Work out the finished part from the listing and answer in its coordinate system (mm). Round coordinates to 2 decimals unless told otherwise and drop trailing zeros. Order: outer loops, then holes, each group sorted by start corner. A loop starts at its lowest first (then second) coordinate and runs counter-clockwise, first axis right, second up. Notation, with made-up numbers: (5, 74.5) - (41, 74.5) arc R14 ccw to (41, 92.5) - close; hole circle Ø9 at (64, -29.5). An arc over 180 degrees is marked (long way). Answer in a Markdown table with one row per item.
Autodesk Inventor part; units mm, degrees
ref_plane "Start Plane" through (0, 0, 19.7356) normal (0, 0, 1) x (1, 0, 0)
ref_plane "End Plane" through (0, 0, 1295.0132) normal (0, 0, 1) x (1, 0, 0)
ref_plane "Work Plane4" through (-472.3083, -9, 221.6126) normal (-0.3985724, 0, -0.9171369) x (-0.9171369, 0, 0.3985724)
ref_plane "Start Plane" through (0, 0, 19.7356) normal (0, 0, 1) x (1, 0, 0)
ref_plane "End Plane" through (0, 0, 1295.0132) normal (0, 0, 1) x (1, 0, 0)
sketch "Sketch" plane through (0, 0, 0) normal (0, 0, 1) x (1, 0, 0)
  line L0 (-15, -9) -> (-15, 9)
  line L1 (-9, 15) -> (9, 15)
  line L2 (15, 9) -> (15, -9)
  line L3 (9, -15) -> (-9, -15)
  arc A0 (-15, -9) -> (-9, -15) centre (-9, -9) ccw
  arc A1 (-9, 15) -> (-15, 9) centre (-9, 9) ccw
  arc A2 (15, 9) -> (9, 15) centre (9, 9) ccw
  arc A3 (9, -15) -> (15, -9) centre (9, -9) ccw
  arc A4 (-9, 12) -> (-12, 9) centre (-9, 9) ccw
  line L4 (-9, 12) -> (9, 12)
  arc A5 (12, 9) -> (9, 12) centre (9, 9) ccw
  line L5 (12, 9) -> (12, -9)
  arc A6 (9, -12) -> (12, -9) centre (9, -9) ccw
  line L6 (9, -12) -> (-9, -12)
  arc A7 (-12, -9) -> (-9, -12) centre (-9, -9) ccw
  line L7 (-12, -9) -> (-12, 9)
  line L8 (0, 22.7397) -> (0, -22.7397) construction
  line L9 (-22.7397, 0) -> (22.7397, 0) construction
  dimension "d7" = 6
  dimension "d10" = 30
  dimension "d11" = 30
  dimension "d12" = 3
  dimension "d15" = 15
  dimension "d16" = 15
extrude "Body" add sketch "Sketch" along normal up to surface (1275.2776 mm away) from surface at 19.7356
sketch "Sketch3" plane through (0, 0, 0) normal (0, 0, 1) x (1, 0, 0)
  line L0 (0, 0) -> (10, 0)
ref_plane "Work Plane3" through (0, 0, 0) normal (0, -1, 0) x (1, 0, 0)
ref_plane "Work Plane4" through (-472.3083, -9, 221.6126) normal (-0.3985724, 0, -0.9171369) x (-0.9171369, 0, 0.3985724)
split "Split1" plane through (-472.3083, -9, 221.6126) removes the side toward (-0.3985724, 0, -0.9171369)
ref_plane "Work Plane5" through (-464.5298, 9, 201.8769) normal (-0.9171369, 0, 0.3985724) x (0.3985724, 0, 0.9171369)
split "Split2" plane through (-464.5298, 9, 201.8769) removes the side toward (-0.9171369, 0, 0.3985724)
ref_plane "Work Plane6" through (1.6776, 9, 1293.5139) normal (-0.1118382, 0, 0.9937264) x (0.9937264, 0, 0.1118382)
split "Split3" plane through (1.6776, 9, 1293.5139) removes the side toward (-0.1118382, 0, 0.9937264)
ref_plane "Work Plane7" through (584.1015, 9, 1381.6839) normal (0.9171369, 0, -0.3985724) x (-0.3985724, 0, -0.9171369)
split "Split4" plane through (584.1015, 9, 1381.6839) removes the side toward (0.9171369, 0, -0.3985724)
sketch "Sketch4" plane through (0, 0, 0) normal (0, -1, 0) x (1, 0, 0)
  line L0 (-2, 19.7356) -> (12, 19.7356)
  line L1 (-2, 1295.0132) -> (12, 1295.0132)
  dimension "d18" = 1275.2776
equation "\"d7\" = G_IR"
equation "\"d10\" = G_H"
equation "\"d11\" = G_W"
equation "\"d12\" = G_T"
equation "\"d15\" = 0.5 * d10"
equation "\"d16\" = 0.5 * d11"
equation "\"d3\" = G_L"
equation "\"G_W\" = 30"
equation "\"G_H\" = 30"
equation "\"G_T\" = 3"
equation "\"G_IR\" = 6"
equation "\"G_L\" = d18"
equation "\"G_OFFSET_START\" = -19.73564"
equation "\"G_OFFSET_END\" = -13.40653"
equation "\"d13\" = -G_OFFSET_START"
equation "\"d14\" = G_OFFSET_END + B_L"
equation "\"B_L\" = 1308.41975"
properties part number "DIN EN 10219-2 - 30 x 30 x 3  - 1275.28" material "Steel, Mild"
1) The mould has two halves that part along X. Classify faces 1 (the face through (4.4, 12.15, 47.76)), 2 (the face through (-4.165, -12.292, 1261.201)): released by +X, released by -X, zero draft, split by the parting line, or undercut.
Filled in:
| item | result |
|---|---|
| face 1 | released by +X |
| face 2 | released by -X |
2) Find section B-B, the plane x = 3.5. Give the vertices of the cut face in (y, z).
Filled in:
| item | result |
|---|---|
| outline | (-15, 45.69) - (-12, 45.69) - (-12, 1278.84) - (-15, 1278.84) - close; (12, 45.69) - (15, 45.69) - (15, 1278.84) - (12, 1278.84) - close |
3) Find the intervals of material crossed by probe 1 along X at (y, z) = (7.5, 950); probe 2 along Y at (x, z) = (11.5, 406.5), in increasing order. Write a range as from..to.
Filled in:
| item | result |
|---|---|
| probe 1 | x = -15..-12, 12..15 |
| probe 2 | y = -14.45..-10.66, 10.66..14.45 |
4) Find section C-C, the plane y = 4.5. Give the vertices of the cut face in (x, z).
Filled in:
| item | result |
|---|---|
| outline | (-15, 22.87) - (-12, 21.57) - (-12, 1243.17) - (-15, 1236.27) - close; (12, 65.25) - (15, 72.15) - (15, 1295.01) - (12, 1294.68) - close |
5) Find section A-A, the plane z = 890.5. Give the vertices of the cut face in (x, y).
Filled in:
| item | result |
|---|---|
| outline | (-15, -9) arc R6 ccw to (-9, -15) - (9, -15) arc R6 ccw to (15, -9) - (15, 9) arc R6 ccw to (9, 15) - (-9, 15) arc R6 ccw to (-15, 9) - close; hole (-12, -9) arc R3 ccw to (-9, -12) - (9, -12) arc R3 ccw to (12, -9) - (12, 9) arc R3 ccw to (9, 12) - (-9, 12) arc R3 ccw to (-12, 9) - close |
